```python
from build123d import *

# Parameters (mm, degrees)
ESQUISSE1_R                                 = 1.6
BOSS_EXTRU_1_DEPTH                          = 2
FRAISAGE_POUR_VIS_T_TE_FRAIS_E_M42_AT_COUNT = 2
FRAISAGE_POUR_VIS_T_TE_FRAIS_E_M42_AT_PITCH = 197.989898732
FRAISAGE_POUR_VIS_T_TE_FRAIS_E_M42_2_COUNT  = 2
FRAISAGE_POUR_VIS_T_TE_FRAIS_E_M42_2_PITCH  = 197.989898732
FRAISAGE_POUR_VIS_T_TE_FRAIS_E_M42_3_COUNT  = 2
FRAISAGE_POUR_VIS_T_TE_FRAIS_E_M42_3_PITCH  = 280


with BuildPart() as part:
    # Esquisse1 → Boss.-Extru.1 (new body)
    with BuildSketch(Plane.XY):
        with BuildLine():
            Line((-74.833147735, 130), (74.833147735, 130))
            ThreePointArc((74.833147735, 130), (123.291527294, 85.435351568), (148, 24.413111231))
            Line((148, 24.413111231), (148, -24.413111231))
            ThreePointArc((148, -24.413111231), (0, -150), (-148, -24.413111231))
            Line((-148, -24.413111231), (-148, 24.413111231))
            ThreePointArc((-148, 24.413111231), (-123.291527294, 85.435351568), (-74.833147735, 130))
        make_face()
        with Locations((-98.994949366, 98.994949366)):
            Circle(ESQUISSE1_R, mode=Mode.SUBTRACT)
        with Locations((-98.994949366, -98.994949366)):
            Circle(ESQUISSE1_R, mode=Mode.SUBTRACT)
        with Locations((98.994949366, -98.994949366)):
            Circle(ESQUISSE1_R, mode=Mode.SUBTRACT)
        with Locations((98.994949366, 98.994949366)):
            Circle(ESQUISSE1_R, mode=Mode.SUBTRACT)
    extrude(amount=BOSS_EXTRU_1_DEPTH)

    # Esquisse4 → Fraisage pour vis à tête fraisée M42 (revolve, cut)
    with BuildSketch(Plane(origin=(98.994949366, 98.994949366, 2), x_dir=(0, -1, 0), z_dir=(1, 0, 0))):
        Polygon((0, 0), (0, 2), (2.25, 2), (2.25, 2.45), (4.7, 0), align=None)
    fraisage_pour_vis_t_te_frais_e_m42 = revolve(axis=Axis((98.994949366, 98.994949366, 8.35), (0, 0, -1)), mode=Mode.SUBTRACT)

    # Fraisage pour vis à tête fraisée M42 at: Fraisage pour vis à tête fraisée M42 ×2
    with Locations(*[(-i * FRAISAGE_POUR_VIS_T_TE_FRAIS_E_M42_AT_PITCH, 0, 0) for i in range(1, FRAISAGE_POUR_VIS_T_TE_FRAIS_E_M42_AT_COUNT)]):
        add(fraisage_pour_vis_t_te_frais_e_m42, mode=Mode.SUBTRACT)

    # Fraisage pour vis _ t_te frais_e M42 2: Fraisage pour vis à tête fraisée M42 ×2
    with Locations(*[(0, -i * FRAISAGE_POUR_VIS_T_TE_FRAIS_E_M42_2_PITCH, 0) for i in range(1, FRAISAGE_POUR_VIS_T_TE_FRAIS_E_M42_2_COUNT)]):
        add(fraisage_pour_vis_t_te_frais_e_m42, mode=Mode.SUBTRACT)

    # Fraisage pour vis _ t_te frais_e M42 3: Fraisage pour vis à tête fraisée M42 ×2
    with Locations(*[Vector(-0.707106781186546, -0.707106781186549, 0) * (i * FRAISAGE_POUR_VIS_T_TE_FRAIS_E_M42_3_PITCH) for i in range(1, FRAISAGE_POUR_VIS_T_TE_FRAIS_E_M42_3_COUNT)]):
        add(fraisage_pour_vis_t_te_frais_e_m42, mode=Mode.SUBTRACT)


solid = part.part
```
For this review, take the finished solid that the model builds, in its own axes (mm). Round coordinates to 2 decimals unless told otherwise and drop trailing zeros. Write each loop counter-clockwise with the first axis right and the second up, starting at its lowest first coordinate (ties: lowest second). Pieces come first, ordered by that corner, then holes. Notation, with made-up numbers: (77.25, -23) - (86.25, -23) arc R24 ccw to (86.25, 13) - close; hole circle Ø5 at (74.5, 40.5). An arc over 180 degrees is marked (long way). Answer as a JSON object with one key per item and string values.
1. For pin 1 Ø1 at (y, z) = (74.5, 0.5) entering from +X; pin 2 Ø1 at (y, z) = (77, 0.5) entering from +X, all flat-tipped, find the tip position at first contact; note any pin that passes through.
Response values:
{"pin 1": "stops at x = 130.48", "pin 2": "stops at x = 129.03"}
2. To check wall thickness, follow line 1 along X through (y, z) = (-102, 1.4); line 2 along X through (y, z) = (119, 1.75); line 3 along X through (y, z) = (-105.5, 1.5). State the ranges of each line that lie inside material, in increasing order.
Response values:
{"line 1": "x = -109.98 to -101.78, -96.21 to 96.21, 101.78 to 109.98", "line 2": "x = -91.32 to 91.32", "line 3": "x = -106.63 to 106.63"}
3. We need section B-B on y = 90. Give the boundary of the cut face in (x, z), then the cut area to 3 significant figures.
Response values:
{"outline": "(-120, 0) - (120, 0) - (120, 2) - (-120, 2) - close", "area": "480 mm2"}
4. We need section C-C on x = -82. Give the boundary of the cut face in (y, z), then the cut area to 3 significant figures.
Response values:
{"outline": "(-125.6, 0) - (125.6, 0) - (125.6, 2) - (-125.6, 2) - close", "area": "502 mm2"}
5. We need section A-A on z = 1.5. Give the boundary of the cut face in (x, y).
Response values:
{"outline": "(-148, -24.41) arc R150 ccw to (148, -24.41) - (148, 24.41) arc R150 ccw to (74.83, 130) - (-74.83, 130) arc R150 ccw to (-148, 24.41) - close; hole circle Ø8.4 at (-98.99, -98.99); hole circle Ø8.4 at (-98.99, 98.99); hole circle Ø8.4 at (98.99, -98.99); hole circle Ø8.4 at (98.99, 98.99)"}
